For this review, take the finished solid that the model builds, in its own axes (mm). A direction names the side the tool comes from. Coordinates: 2 decimals unless noted, no trailing zeros. Write each loop counter-clockwise with the first axis right and the second up, starting at its lowest first coordinate (ties: lowest second). Pieces come first, ordered by that corner, then holes.
Autodesk Inventor part; units mm, degrees
ref_plane "YZ Plane" through (0, 0, 0) normal (1, 0, 0) x (0, 1, 0)
ref_plane "XZ Plane" through (0, 0, 0) normal (0, 1, 0) x (-1, 0, 0)
ref_plane "XY Plane" through (0, 0, 0) normal (0, 0, 1) x (1, 0, 0)
sketch "Sketch3" plane through (0, 0, 0) normal (0, 1, 0) x (-1, 0, 0)
  line L0 (0, 0) -> (0, -60)
  line L1 (0, 0) -> (60, 0) construction
  line L2 (0, -60) -> (12.519, -60)
  line L3 (0, 0) -> (41, 0)
  line L4 (41, 0) -> (41, 7.5)
  line L5 (41, 7.5) -> (56, 7.5)
  circle A0 centre (48.5, 7.5) radius 7.5
  circle A1 centre (48.5, 7.5) radius 3
  line L6 (56, 7.5) -> (56, -16.519)
  line L7 (56, -16.519) -> (12.519, -60)
  line L8 (0, -30) -> (5, -30)
  line L9 (5, -60) -> (5, -48)
  line L10 (5, 0) -> (5, -12)
  circle A2 centre (5, -12) radius 1.5
  circle A3 centre (5, -48) radius 1.5
  dimension "d6" = 60
  dimension "d7" = 90
  dimension "d8" = 12.519
  dimension "d9" = 41
  dimension "d10" = 7.5
  dimension "d11" = 15
  dimension "d12" = 6
  dimension "d13" = 24.019
  dimension "d18" = 5
  dimension "d19" = 12
  dimension "d20" = 12
  dimension "d21" = 3
  dimension "d22" = 3
extrude "Extrusion1" add sketch "Sketch3" along normal blind 3 contours L3 L4 A0 L6 L7 L2 L0 | A0 L5 A1 | L5 A1 A0 | L5 A1 picked at (49.4145, 6.796)
sketch "Sketch4" plane through (0, 0, 0) normal (0, -1, 0) x (1, 0, 0)
  line L0 (-51.5, 7.5) -> (-45.5, 7.5)
  line L1 (-45.5, 7.5) -> (-51.5, 7.5)
  circle A0 centre (-48.5, 7.5) radius 3
  point P0 (0, 0)
extrude "Extrusion2" add sketch "Sketch4" against normal blind 8
properties part number "sideplateshaft_std"
Q1. Add section B-B (x = -48.5). State the section outline as (y, z) points, then the cut area to 3 significant figures.
Ans:
outline: (0, -24.02) - (3, -24.02) - (3, 4.5) - (8, 4.5) - (8, 10.5) - (3, 10.5) - (3, 15) - (0, 15) - close
area: 147 mm2
Q2. Clearance check with flat-ended pins moving along their axes: pin 1 Ø2 at (x, z) = (-36.5, -6.5) entering from +Y; pin 2 Ø0.9 at (y, z) = (1.5, 3.5) entering from +X; pin 3 Ø0.9 at (x, y) = (-14, 2) entering from +Z. State where each tip first meets the part, or that it passes through.
Ans:
pin 1: stops at y = 3
pin 2: stops at x = -41
pin 3: stops at z = 0
Q3. Draft analysis for pull direction X (two halves, no side actions). For faces 4 (the cylindrical face through (-6.386, 1.479, -11.425)), 5 (the cylindrical face through (-48.34, 1.48, 15)), 6 (the flat face through (-21, 3, -22)), state which applies: +X half, -X half, draft (parallel to the pull), parting line (faces both ways), or undercut.
Ans:
face 4: undercut
face 5: parting line
face 6: draft
Q4. Tool access review of faces 1 (the cylindrical face through (-51.5, 5.5, 7.6)), 2 (the flat face through (-56, 1, -4)), 3 (the flat face through (-20, 1, 0)): name each direction out of +Z, -Z, +X, -X, +Y, -Y from which nothing blocks a thin tool from reaching the whole face with its end or side.
Ans:
face 1: +Y
face 2: +Z, -Z, -X, +Y, -Y
face 3: +Z, +X, +Y, -Y
Q5. Add section A-A (z = -12). State the section outline as (x, y) points.
Ans:
outline: (-56, 0) - (-6.5, 0) - (-6.5, 3) - (-56, 3) - close; (-3.5, 0) - (0, 0) - (0, 3) - (-3.5, 3) - close
Q6. For probe 1 along Z at (x, y) = (-5, 0.85); probe 2 along Y at (x, z) = (-31, -40.5); probe 3 along X at (y, z) = (2.2, -48), list the stretches that pass through material, from the lowest coordinate up.
Ans:
probe 1: z = -60 to -49.5, -46.5 to -13.5, -10.5 to 0
probe 2: y = 0 to 3
probe 3: x = -24.52 to -6.5, -3.5 to 0
Q7. Add section C-C (y = 5.25). State the section outline as (x, z) points, then the cut area to 3 significant figures.
Ans:
outline: circle Ø6 at (-48.5, 7.5)
area: 28.3 mm2
Q8. Add section D-D (z = -48). State the section outline as (x, y) points.
Ans:
outline: (-24.52, 0) - (-6.5, 0) - (-6.5, 3) - (-24.52, 3) - close; (-3.5, 0) - (0, 0) - (0, 3) - (-3.5, 3) - close
